Verification items for this drawing (mm, ordinates from the low corner). A direction names the side the tool comes from. Round coordinates to 2 decimals unless told otherwise and drop trailing zeros. Order: outer loops, then holes, each group sorted by start corner. A loop starts at its lowest first (then second) coordinate and runs counter-clockwise, first axis right, second up. Notation, with made-up numbers: (18.25, 0.5) -> (60.25, 0.5) arc R11 cw to (60.25, 7.5) -> close; hole circle Ø7 at (41, -38.5). An arc over 180 degrees is marked (long way). Answer in a Markdown table with one row per item. Add a question column.
1. Material ranges on L1, parallel to X at y = 20, z = 82 (1 decimal); L2, parallel to Z at x = 30, y = 22; L3, parallel to Y at x = 8.5, z = 47, recorded low to high. Write a range as from..to.
2. Draft check along Z on the marked faces 1, 2, 3 and 4. Enter one of: +Z half, -Z half, draft (parallel to the pull), parting line (faces both ways), or undercut.
3. Depth check by flat-ended pin: P1, Ø3, axis at x = 7.5, y = 7.5, coming from the +Z side; P2, Ø6, axis at y = 8.5, z = 122, coming from the -X side (1 decimal); P3, Ø6.5, axis at x = 59, z = 51, coming from the -Y side; P4, Ø1, axis at x = 53, y = 5, coming from the -Z side. Enter the tip coordinate at first touch or a pass-through.
4. Sectioned sample at B-B, the plane x = 22. Record the boundary of the cut face in (y, z).
5. Access from +Z, -Z, +X, -X, +Y, -Y to the whole of each face (thin tool, end or side, straight path). Record for the marked faces 5, 6 and 7.
6. Sectioned sample at C-C, the plane y = 29.5. Record the boundary of the cut face in (x, z) (1 decimal), then the cut area to 3 significant figures.
7. Sectioned sample at A-A, the plane z = 113.5. Record the boundary of the cut face in (x, y) (1 decimal).
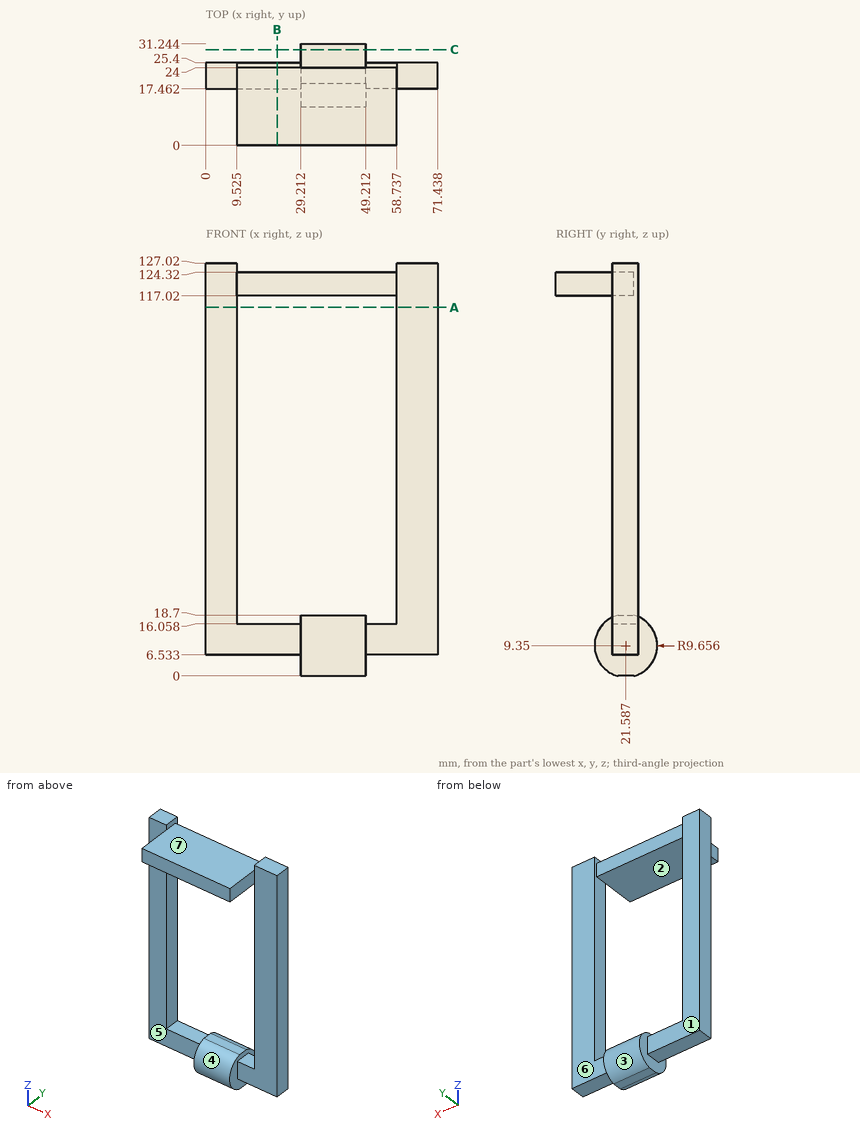
Answer key:
| question | item | result |
|---|---|---|
| 1 | L1 | x = 0..9.5, 58.7..71.4 |
| 1 | L2 | z = 0..18.7, 117.02..124.32 |
| 1 | L3 | y = 17.46..25.4 |
| 2 | face 1 | draft |
| 2 | face 2 | undercut |
| 2 | face 3 | parting line |
| 2 | face 4 | undercut |
| 3 | P1 | passes through |
| 3 | P2 | stops at x = 9.5 |
| 3 | P3 | stops at y = 17.46 |
| 3 | P4 | stops at z = 117.02 |
| 4 | outline | (0, 117.02) -> (24, 117.02) -> (24, 124.32) -> (0, 124.32) -> close; (17.46, 6.53) -> (25.4, 6.53) -> (25.4, 16.06) -> (17.46, 16.06) -> close |
| 5 | face 5 | -Z, -X, -Y |
| 5 | face 6 | +Z, -Z, +X, +Y |
| 5 | face 7 | +Z, +Y, -Y |
| 6 | outline | (29.2, 3.8) -> (49.2, 3.8) -> (49.2, 14.9) -> (29.2, 14.9) -> close |
| 6 | area | 221 mm² |
| 7 | outline | (0, 17.5) -> (9.5, 17.5) -> (9.5, 25.4) -> (0, 25.4) -> close; (58.7, 17.5) -> (71.4, 17.5) -> (71.4, 25.4) -> (58.7, 25.4) -> close |
